Part model, mm, in its own coordinate system. A direction names the side the tool comes from. Coordinates: 2 decimals unless noted, no trailing zeros. Loops run counter-clockwise (first coordinate to the right, second up) from the corner with the lowest first, then second, coordinate; pieces in that order, holes last. Notation, with made-up numbers: M -28.5,46.25 L 20.5,46.25 A27 ccw 20.5,81.25 Z; hole C -1.75,-35 d9. An arc over 180 degrees is marked long. Use a Markdown table: item, result. Add a question column.
1) Band-saw the part on D-D (z = 8). List the corners of the cut face in (x, y).
2) Band-saw the part on B-B (z = -21). State how many separate pieces and enclosed holes the cut face has, plus the area to 3 significant figures.
3) Pull direction Y, two halves, no side cores. Call faces 1 (the flat face through (-7.113, -23, -6)), 2 (the flat face through (17, 27, -10)), 3 (the flat face through (35.8, -7.5, 3.8)): released by +Y, released by -Y, zero draft, split by the parting line, or undercut.
4) Tool access for faces 4 (the flat face through (-37, 29, -10)), 5 (the flat face through (37, -30, -21)), 6 (the flat face through (12, -12, -1)), 7 (the flat face through (37, -28.5, -11)), 8 (the flat face through (45, 26, -14)): list every direction of +Z, -Z, +X, -X, +Y, -Y with a clear straight run to the whole face (end or side of a thin tool).
5) Pin check, flat tips, straight feed: pin 1 Ø12 at (x, z) = (-25.5, 2) entering from +Y; pin 2 Ø1.5 at (x, y) = (44.5, 29.5) entering from -Z; pin 3 Ø4.5 at (y, z) = (19, -7.5) entering from +X. Stop position of each tip, or through.
6) Wall check: probe 1 along Y at (x, z) = (7, -1.2); probe 2 along Y at (x, z) = (44.7, -22.35); probe 3 along Y at (x, z) = (41, -15). Give the ranges that are in metal, low to high. Write a range as from..to.
7) Band-saw the part on A-A (y = 29.7). List the corners of the cut face in (x, z), plus the area to 3 significant figures.
8) Band-saw the part on C-C (x = -11.5). List the corners of the cut face in (y, z), plus the area to 4 significant figures.
from build123d import *

# Parameters (mm, degrees)
SKETCH_1_W           = 94
SKETCH_1_H           = 64
EXTRUDE_1_DEPTH      = 25
SKETCH_3_W           = 86
SKETCH_3_H           = 57
CUT_EXTRUDE_1_DEPTH  = 23
FILLET_1_R           = 1
SKETCH_4_W           = 77
SKETCH_4_H           = 10
CUT_EXTRUDE_3_DEPTH  = 5
FILLET_4_R           = 1
SKETCH_5_W           = 54
SKETCH_5_H           = 25
CUT_EXTRUDE_4_DEPTH  = 12
SKETCH_6_W           = 30
SKETCH_6_H           = 20
CUT_EXTRUDE_5_DEPTH  = 18
SKETCH_7_W           = 22
SKETCH_7_H           = 52
CUT_EXTRUDE_6_DEPTH  = 5
SKETCH_8_W           = 30.5
SKETCH_8_H           = 30.5
CUT_EXTRUDE_7_DEPTH  = 5
FILLET_5_R           = 1
SKETCH_9_R           = 1.55
CUT_EXTRUDE_8_DEPTH  = 5
SKETCH_10_W          = 4
SKETCH_10_H          = 53.4
CUT_EXTRUDE_9_DEPTH  = 22
SKETCH_11_W          = 30.5
SKETCH_11_H          = 11.890365251
EXTRUDE_2_DEPTH      = 9
SKETCH_12_W          = 54.61329803
SKETCH_12_H          = 6.109634749
SKETCH_12_W_2        = 5.38670197
SKETCH_12_H_2        = 57
SKETCH_12_W_3        = 8
SKETCH_12_H_3        = 27
EXTRUDE_3_DEPTH      = 9
SKETCH_13_R          = 2
CUT_EXTRUDE_10_DEPTH = 10
SKETCH_14_W          = 15
SKETCH_14_H          = 15
EXTRUDE_4_DEPTH      = 14
SKETCH_17_R          = 4
CUT_EXTRUDE_13_DEPTH = 67.289139382
FILLET_7_R           = 4
SKETCH_18_W          = 15
SKETCH_18_H          = 5
CUT_EXTRUDE_14_DEPTH = 63.112800613


with BuildPart() as part:
    # 草图1 → 凸台-拉伸1 (new body)
    with BuildSketch(Plane.XY):
        Rectangle(SKETCH_1_W, SKETCH_1_H)
    extrude(amount=-EXTRUDE_1_DEPTH)

    # 草图3 → 切除-拉伸1 (cut)
    with BuildSketch(Plane(origin=(0, 0, -25), x_dir=(-1, 0, 0), z_dir=(0, 0, -1))):
        Rectangle(SKETCH_3_W, SKETCH_3_H)
    extrude(amount=-CUT_EXTRUDE_1_DEPTH, mode=Mode.SUBTRACT)

    # 圆角1
    fillet_1_edges = [part.edges().sort_by_distance(p)[0] for p in [
        (47, -32, -12.5),
        (-47, -32, -12.5),
        (-47, 32, -12.5),
        (47, 32, -12.5),
    ]]
    fillet(fillet_1_edges, radius=FILLET_1_R)

    # 草图4 → 切除-拉伸3 (cut)
    with BuildSketch(Plane.XZ.offset(32)):
        with Locations((-1.5, -20)):
            Rectangle(SKETCH_4_W, SKETCH_4_H)
    extrude(amount=-CUT_EXTRUDE_3_DEPTH, mode=Mode.SUBTRACT)

    # 圆角4
    fillet_4_edges = [part.edges().sort_by_distance(p)[0] for p in [
        (37, -30.25, -15),
        (-40, -30.25, -15),
    ]]
    fillet(fillet_4_edges, radius=FILLET_4_R)

    # 草图5 → 切除-拉伸4 (cut)
    with BuildSketch(Plane(origin=(0, 32, 0), x_dir=(1, 0, 0), z_dir=(0, 1, 0))):
        with Locations((-10, 12.5)):
            Rectangle(SKETCH_5_W, SKETCH_5_H)
    extrude(amount=-CUT_EXTRUDE_4_DEPTH, mode=Mode.SUBTRACT)

    # 草图6 → 切除-拉伸5 (cut)
    with BuildSketch(Plane.XY):
        with Locations((12, -22)):
            Rectangle(SKETCH_6_W, SKETCH_6_H)
    extrude(amount=-CUT_EXTRUDE_5_DEPTH, mode=Mode.SUBTRACT)

    # 草图7 → 切除-拉伸6 (cut)
    with BuildSketch(Plane.ZY.offset(47)):
        with Locations((-14, 0)):
            Rectangle(SKETCH_7_W, SKETCH_7_H)
    extrude(amount=-CUT_EXTRUDE_6_DEPTH, mode=Mode.SUBTRACT)

    # 草图8 → 切除-拉伸7 (cut)
    with BuildSketch(Plane.XY):
        with Locations((-22.36329803, -1.359634749)):
            Rectangle(SKETCH_8_W, SKETCH_8_H)
    extrude(amount=-CUT_EXTRUDE_7_DEPTH, mode=Mode.SUBTRACT)

    # 圆角5
    fillet_5_edges = [part.edges().sort_by_distance(p)[0] for p in [
        (-7.11329803, 13.890365251, -1),
        (-7.11329803, -16.609634749, -1),
        (-37.61329803, -16.609634749, -1),
        (-37.61329803, 13.890365251, -1),
    ]]
    fillet(fillet_5_edges, radius=FILLET_5_R)

    # 草图9 → 切除-拉伸8 (cut)
    with BuildSketch(Plane(origin=(0, 0, -25), x_dir=(-1, 0, 0), z_dir=(0, 0, -1))):
        with Locations((44.7, 29.7)):
            Circle(SKETCH_9_R)
        with Locations(Location((44.7, -29.7, 0), (0, 0, 180))):
            Circle(SKETCH_9_R)
        with Locations((-44.7, -29.7)):
            Circle(SKETCH_9_R)
        with Locations(Location((-44.7, 29.7, 0), (0, 0, 180))):
            Circle(SKETCH_9_R)
    extrude(amount=-CUT_EXTRUDE_8_DEPTH, mode=Mode.SUBTRACT)

    # 草图10 → 切除-拉伸9 (cut)
    with BuildSketch(Plane(origin=(0, 0, -25), x_dir=(-1, 0, 0), z_dir=(0, 0, -1))):
        with Locations((-45, -0.7)):
            Rectangle(SKETCH_10_W, SKETCH_10_H)
    extrude(amount=-CUT_EXTRUDE_9_DEPTH, mode=Mode.SUBTRACT)

    # 草图11 → 凸台-拉伸2 (add)
    with BuildSketch(Plane(origin=(0, 0, -2), x_dir=(-1, 0, 0), z_dir=(0, 0, -1))):
        with Locations((22.36329803, -22.554817375)):
            Rectangle(SKETCH_11_W, SKETCH_11_H)
    extrude(amount=EXTRUDE_2_DEPTH)

    # 草图12 → 凸台-拉伸3 (add)
    with BuildSketch(Plane(origin=(0, 0, -2), x_dir=(-1, 0, 0), z_dir=(0, 0, -1))):
        with Locations((10.306649015, 16.945182625)):
            Rectangle(SKETCH_12_W, SKETCH_12_H)
        with Locations((40.306649015, 0)):
            Rectangle(SKETCH_12_W_2, SKETCH_12_H_2)
        with Locations((-21, 15)):
            Rectangle(SKETCH_12_W_3, SKETCH_12_H_3)
    extrude(amount=EXTRUDE_3_DEPTH)

    # 草图13 → 切除-拉伸10 (cut)
    with BuildSketch(Plane.XY):
        with Locations((0, 10.839030868)):
            Circle(SKETCH_13_R)
        with Locations((7, 10.839030868)):
            Circle(SKETCH_13_R)
        with Locations((14, 10.839030868)):
            Circle(SKETCH_13_R)
        with Locations((7, 1.839030868)):
            Circle(SKETCH_13_R)
        with Locations((14, 1.839030868)):
            Circle(SKETCH_13_R)
        with Locations((7, -7.160969132)):
            Circle(SKETCH_13_R)
        with Locations((14, -7.160969132)):
            Circle(SKETCH_13_R)
        with Locations((0, 1.839030868)):
            Circle(SKETCH_13_R)
        with Locations((0, -7.160969132)):
            Circle(SKETCH_13_R)
    extrude(amount=-CUT_EXTRUDE_10_DEPTH, mode=Mode.SUBTRACT)

    # 草图14 → 凸台-拉伸4 (add)
    with BuildSketch(Plane.XY):
        with Locations((35.885750834, 0)):
            Rectangle(SKETCH_14_W, SKETCH_14_H)
    extrude(amount=EXTRUDE_4_DEPTH)

    # 草图17 → 切除-拉伸13 (cut, through all)
    with BuildSketch(Plane.XZ.offset(7.5)):
        with Locations(Location((35.885750834, 8, 0), (0, 0, 270))):
            Circle(SKETCH_17_R)
    extrude(amount=-CUT_EXTRUDE_13_DEPTH, mode=Mode.SUBTRACT)

    # 圆角7
    fillet_7_edges = [part.edges().sort_by_distance(p)[0] for p in [
        (43.385750834, 0, 14),
        (28.385750834, 0, 14),
    ]]
    fillet(fillet_7_edges, radius=FILLET_7_R)

    # 草图18 → 切除-拉伸14 (cut, through all)
    with BuildSketch(Plane.XY):
        with Locations((35.885750834, 0)):
            Rectangle(SKETCH_18_W, SKETCH_18_H)
    extrude(amount=CUT_EXTRUDE_14_DEPTH, mode=Mode.SUBTRACT)


solid = part.part
Entries:
| question | item | result |
|---|---|---|
| 1 | outline | M 28.39,-7.5 L 31.89,-7.5 L 31.89,-2.5 L 28.39,-2.5 Z; M 28.39,2.5 L 31.89,2.5 L 31.89,7.5 L 28.39,7.5 Z; M 39.89,-7.5 L 43.39,-7.5 L 43.39,-2.5 L 39.89,-2.5 Z; M 39.89,2.5 L 43.39,2.5 L 43.39,7.5 L 39.89,7.5 Z |
| 2 | separate pieces | 4 |
| 2 | enclosed holes | 4 |
| 2 | area | 203 mm2 |
| 3 | face 1 | undercut |
| 3 | face 2 | zero draft |
| 3 | face 3 | released by -Y |
| 4 | face 4 | +Z, -Z, +Y |
| 4 | face 5 | -Z, -Y |
| 4 | face 6 | +Z, -Z, -Y |
| 4 | face 7 | -Z |
| 4 | face 8 | -Z, +X |
| 5 | pin 1 | y = 20 |
| 5 | pin 2 | z = -20 |
| 5 | pin 3 | x = 25 |
| 6 | probe 1 | -12..-9.16, -5.16..-0.16, 3.84..8.84, 12.84..20 |
| 6 | probe 2 | -32..-31.25, -28.15..-27.4, 26..28.15, 31.25..32 |
| 6 | probe 3 | -32..-28.5, 28.5..32 |
| 7 | outline | M -47,-25 L -46.25,-25 L -46.25,-20 L -43.15,-20 L -43.15,-25 L -37,-25 L -37,0 L -47,0 Z; M 17,-25 L 43.15,-25 L 43.15,-20 L 46.25,-20 L 46.25,-25 L 47,-25 L 47,0 L 17,0 Z |
| 7 | area | 969 mm2 |
| 8 | outline | M -32,-15 L -28.5,-15 L -28.5,-11 L -16.61,-11 L -16.61,0 L -32,0 Z; M 13.89,-11 L 20,-11 L 20,0 L 13.89,0 Z |
| 8 | area | 250.5 mm2 |
